Geometry check sheet. Reference: the model listing, model coordinates, mm. Round coordinates to 2 decimals unless told otherwise and drop trailing zeros.
```python
from build123d import *

# Parameters (mm, degrees)
SKETCH1_R           = 3.4
BOSS_EXTRUDE1_DEPTH = 713
SKETCH2_W           = 40
SKETCH2_H           = 163
CUT_EXTRUDE1_DEPTH  = 715.401147815


with BuildPart() as part:
    # Sketch1 → Boss-Extrude1 (new body)
    with BuildSketch(Plane.XY):
        with BuildLine():
            Line((20, 17.75), (20, 5.15))
            Line((20, 5.15), (19, 5.15))
            Line((19, 5.15), (19, 4.15))
            Line((19, 4.15), (15.4, 4.15))
            Line((15.4, 4.15), (15.4, 6.35))
            Line((15.4, 6.35), (16.95, 6.35))
            ThreePointArc((16.95, 6.35), (17.833883476, 6.716116524), (18.2, 7.6))
            Line((18.2, 7.6), (18.2, 9.3))
            ThreePointArc((18.2, 9.3), (17.907106781, 10.007106781), (17.2, 10.3))
            Line((17.2, 10.3), (12.03669957, 10.3))
            ThreePointArc((12.03669957, 10.3), (11.73040037, 10.239040459), (11.470780817, 10.065452001))
            Line((11.470780817, 10.065452001), (6.084081247, 4.674305984))
            ThreePointArc((6.084081247, 4.674305984), (5.910833239, 4.414848262), (5.85, 4.108853983))
            Line((5.85, 4.108853983), (5.85, -4.108853983))
            ThreePointArc((5.85, -4.108853983), (5.910833239, -4.414848262), (6.084081247, -4.674305984))
            Line((6.084081247, -4.674305984), (11.470780817, -10.065452001))
            ThreePointArc((11.470780817, -10.065452001), (11.73040037, -10.239040459), (12.03669957, -10.3))
            Line((12.03669957, -10.3), (17.2, -10.3))
            ThreePointArc((17.2, -10.3), (17.907106781, -10.007106781), (18.2, -9.3))
            Line((18.2, -9.3), (18.2, -7.6))
            ThreePointArc((18.2, -7.6), (17.833883476, -6.716116524), (16.95, -6.35))
            Line((16.95, -6.35), (15.4, -6.35))
            Line((15.4, -6.35), (15.4, -4.15))
            Line((15.4, -4.15), (19, -4.15))
            Line((19, -4.15), (19, -5.15))
            Line((19, -5.15), (20, -5.15))
            Line((20, -5.15), (20, -17.75))
            ThreePointArc((20, -17.75), (19.340990258, -19.340990258), (17.75, -20))
            Line((17.75, -20), (5.15, -20))
            Line((5.15, -20), (5.15, -19))
            Line((5.15, -19), (4.15, -19))
            Line((4.15, -19), (4.15, -15.4))
            Line((4.15, -15.4), (6.35, -15.4))
            Line((6.35, -15.4), (6.35, -16.95))
            ThreePointArc((6.35, -16.95), (6.716116524, -17.833883476), (7.6, -18.2))
            Line((7.6, -18.2), (9.3, -18.2))
            ThreePointArc((9.3, -18.2), (10.007106781, -17.907106781), (10.3, -17.2))
            Line((10.3, -17.2), (10.3, -12.054477022))
            ThreePointArc((10.3, -12.054477022), (10.239166761, -11.748482743), (10.065918753, -11.489025021))
            Line((10.065918753, -11.489025021), (4.665899173, -6.084547999))
            ThreePointArc((4.665899173, -6.084547999), (4.406279619, -5.910959541), (4.09998042, -5.85))
            Line((4.09998042, -5.85), (-4.09998042, -5.85))
            ThreePointArc((-4.09998042, -5.85), (-4.406279619, -5.910959541), (-4.665899173, -6.084547999))
            Line((-4.665899173, -6.084547999), (-10.065918753, -11.489025021))
            ThreePointArc((-10.065918753, -11.489025021), (-10.239166761, -11.748482743), (-10.3, -12.054477022))
            Line((-10.3, -12.054477022), (-10.3, -17.2))
            ThreePointArc((-10.3, -17.2), (-10.007106781, -17.907106781), (-9.3, -18.2))
            Line((-9.3, -18.2), (-7.6, -18.2))
            ThreePointArc((-7.6, -18.2), (-6.716116524, -17.833883476), (-6.35, -16.95))
            Line((-6.35, -16.95), (-6.35, -15.4))
            Line((-6.35, -15.4), (-4.15, -15.4))
            Line((-4.15, -15.4), (-4.15, -19))
            Line((-4.15, -19), (-5.15, -19))
            Line((-5.15, -19), (-5.15, -20))
            Line((-5.15, -20), (-17.75, -20))
            ThreePointArc((-17.75, -20), (-19.340990258, -19.340990258), (-20, -17.75))
            Line((-20, -17.75), (-20, -5.15))
            Line((-20, -5.15), (-19, -5.15))
            Line((-19, -5.15), (-19, -4.15))
            Line((-19, -4.15), (-15.4, -4.15))
            Line((-15.4, -4.15), (-15.4, -6.35))
            Line((-15.4, -6.35), (-16.95, -6.35))
            ThreePointArc((-16.95, -6.35), (-17.833883476, -6.716116524), (-18.2, -7.6))
            Line((-18.2, -7.6), (-18.2, -9.3))
            ThreePointArc((-18.2, -9.3), (-17.907106781, -10.007106781), (-17.2, -10.3))
            Line((-17.2, -10.3), (-12.03669957, -10.3))
            ThreePointArc((-12.03669957, -10.3), (-11.73040037, -10.239040459), (-11.470780817, -10.065452001))
            Line((-11.470780817, -10.065452001), (-6.084081247, -4.674305984))
            ThreePointArc((-6.084081247, -4.674305984), (-5.910833239, -4.414848262), (-5.85, -4.108853983))
            Line((-5.85, -4.108853983), (-5.85, 4.108853983))
            ThreePointArc((-5.85, 4.108853983), (-5.910833239, 4.414848262), (-6.084081247, 4.674305984))
            Line((-6.084081247, 4.674305984), (-11.470780817, 10.065452001))
            ThreePointArc((-11.470780817, 10.065452001), (-11.73040037, 10.239040459), (-12.03669957, 10.3))
            Line((-12.03669957, 10.3), (-17.2, 10.3))
            ThreePointArc((-17.2, 10.3), (-17.907106781, 10.007106781), (-18.2, 9.3))
            Line((-18.2, 9.3), (-18.2, 7.6))
            ThreePointArc((-18.2, 7.6), (-17.833883476, 6.716116524), (-16.95, 6.35))
            Line((-16.95, 6.35), (-15.4, 6.35))
            Line((-15.4, 6.35), (-15.4, 4.15))
            Line((-15.4, 4.15), (-19, 4.15))
            Line((-19, 4.15), (-19, 5.15))
            Line((-19, 5.15), (-20, 5.15))
            Line((-20, 5.15), (-20, 17.75))
            ThreePointArc((-20, 17.75), (-19.340990258, 19.340990258), (-17.75, 20))
            Line((-17.75, 20), (-5.15, 20))
            Line((-5.15, 20), (-5.15, 19))
            Line((-5.15, 19), (-4.15, 19))
            Line((-4.15, 19), (-4.15, 15.4))
            Line((-4.15, 15.4), (-6.35, 15.4))
            Line((-6.35, 15.4), (-6.35, 16.95))
            ThreePointArc((-6.35, 16.95), (-6.716116524, 17.833883476), (-7.6, 18.2))
            Line((-7.6, 18.2), (-9.3, 18.2))
            ThreePointArc((-9.3, 18.2), (-10.007106781, 17.907106781), (-10.3, 17.2))
            Line((-10.3, 17.2), (-10.3, 12.054477022))
            ThreePointArc((-10.3, 12.054477022), (-10.239166761, 11.748482743), (-10.065918753, 11.489025021))
            Line((-10.065918753, 11.489025021), (-4.665899173, 6.084547999))
            ThreePointArc((-4.665899173, 6.084547999), (-4.406279619, 5.910959541), (-4.09998042, 5.85))
            Line((-4.09998042, 5.85), (4.09998042, 5.85))
            ThreePointArc((4.09998042, 5.85), (4.406279619, 5.910959541), (4.665899173, 6.084547999))
            Line((4.665899173, 6.084547999), (10.065918753, 11.489025021))
            ThreePointArc((10.065918753, 11.489025021), (10.239166761, 11.748482743), (10.3, 12.054477022))
            Line((10.3, 12.054477022), (10.3, 17.2))
            ThreePointArc((10.3, 17.2), (10.007106781, 17.907106781), (9.3, 18.2))
            Line((9.3, 18.2), (7.6, 18.2))
            ThreePointArc((7.6, 18.2), (6.716116524, 17.833883476), (6.35, 16.95))
            Line((6.35, 16.95), (6.35, 15.4))
            Line((6.35, 15.4), (4.15, 15.4))
            Line((4.15, 15.4), (4.15, 19))
            Line((4.15, 19), (5.15, 19))
            Line((5.15, 19), (5.15, 20))
            Line((5.15, 20), (17.75, 20))
            ThreePointArc((17.75, 20), (19.340990258, 19.340990258), (20, 17.75))
        make_face()
        with Locations(Location((0, 0, 0), (0, 0, 180))):
            Circle(SKETCH1_R, mode=Mode.SUBTRACT)
        with BuildLine():
            Line((18.6, 16.35), (18.6, 12.2))
            ThreePointArc((18.6, 12.2), (18.365685425, 11.634314575), (17.8, 11.4))
            Line((17.8, 11.4), (12.2, 11.4))
            ThreePointArc((12.2, 11.4), (11.634314575, 11.634314575), (11.4, 12.2))
            Line((11.4, 12.2), (11.4, 17.8))
            ThreePointArc((11.4, 17.8), (11.634314575, 18.365685425), (12.2, 18.6))
            Line((12.2, 18.6), (16.35, 18.6))
            ThreePointArc((16.35, 18.6), (17.940990258, 17.940990258), (18.6, 16.35))
        make_face(mode=Mode.SUBTRACT)
        with BuildLine():
            Line((-12.2, 18.6), (-16.35, 18.6))
            ThreePointArc((-16.35, 18.6), (-17.940990258, 17.940990258), (-18.6, 16.35))
            Line((-18.6, 16.35), (-18.6, 12.2))
            ThreePointArc((-18.6, 12.2), (-18.365685425, 11.634314575), (-17.8, 11.4))
            Line((-17.8, 11.4), (-12.2, 11.4))
            ThreePointArc((-12.2, 11.4), (-11.634314575, 11.634314575), (-11.4, 12.2))
            Line((-11.4, 12.2), (-11.4, 17.8))
            ThreePointArc((-11.4, 17.8), (-11.634314575, 18.365685425), (-12.2, 18.6))
        make_face(mode=Mode.SUBTRACT)
        with BuildLine():
            Line((-18.6, -16.35), (-18.6, -12.2))
            ThreePointArc((-18.6, -12.2), (-18.365685425, -11.634314575), (-17.8, -11.4))
            Line((-17.8, -11.4), (-12.2, -11.4))
            ThreePointArc((-12.2, -11.4), (-11.634314575, -11.634314575), (-11.4, -12.2))
            Line((-11.4, -12.2), (-11.4, -17.8))
            ThreePointArc((-11.4, -17.8), (-11.634314575, -18.365685425), (-12.2, -18.6))
            Line((-12.2, -18.6), (-16.35, -18.6))
            ThreePointArc((-16.35, -18.6), (-17.940990258, -17.940990258), (-18.6, -16.35))
        make_face(mode=Mode.SUBTRACT)
        with BuildLine():
            Line((12.2, -18.6), (16.35, -18.6))
            ThreePointArc((16.35, -18.6), (17.940990258, -17.940990258), (18.6, -16.35))
            Line((18.6, -16.35), (18.6, -12.2))
            ThreePointArc((18.6, -12.2), (18.365685425, -11.634314575), (17.8, -11.4))
            Line((17.8, -11.4), (12.2, -11.4))
            ThreePointArc((12.2, -11.4), (11.634314575, -11.634314575), (11.4, -12.2))
            Line((11.4, -12.2), (11.4, -17.8))
            ThreePointArc((11.4, -17.8), (11.634314575, -18.365685425), (12.2, -18.6))
        make_face(mode=Mode.SUBTRACT)
    extrude(amount=BOSS_EXTRUDE1_DEPTH)

    # Sketch2 → Cut-Extrude1 (cut, through all)
    with BuildSketch(Plane(origin=(0, 20, 0), x_dir=(1, 0, 0), z_dir=(0, 1, 0))):
        with Locations((0, -631.5)):
            Rectangle(SKETCH2_W, SKETCH2_H)
    extrude(amount=-CUT_EXTRUDE1_DEPTH, mode=Mode.SUBTRACT)


solid = part.part
```
(1) Sectioned sample at A-A, the plane z = 355.5. Give the number of separate pieces and of enclosed holes in the cut face, and give its area (3 significant figures).
Returned:
separate pieces: 1
enclosed holes: 5
area: 464 mm2
(2) Depth check by flat-ended pin: P1, Ø0.5, axis at y = -4.5, z = 292.5, coming from the +X side; P2, Ø12, axis at y = -2, z = 130.5, coming from the +X side; P3, Ø0.8, axis at y = 19.5, z = 272.5, coming from the +X side; P4, Ø0.8, axis at x = -19.5, z = 148.5, coming from the +Y side. Enter the tip coordinate at first touch or a pass-through.
Returned:
P1: stops at x = 19
P2: stops at x = 20
P3: stops at x = 19.55
P4: stops at y = 19.55
(3) Material ranges on line 1 (Y direction, x = 5, z = 227); line 2 (X direction, y = 9, z = 122.5); line 3 (Y direction, x = -13, z = 408.5), recorded low to high.
Returned:
line 1: y = -19 to -15.4, -6.42 to 6.42, 15.4 to 19
line 2: x = -20 to -18.2, -10.41 to -7.58, 7.58 to 10.41, 18.2 to 20
line 3: y = -20 to -18.6, -11.4 to -10.3, 10.3 to 11.4, 18.6 to 20
